Work out the finished part from the listing and answer in its coordinate system (mm). Face numbers are marked on the shaded views. A direction names the side the tool comes from. Round coordinates to 2 decimals unless told otherwise and drop trailing zeros. Write each loop counter-clockwise with the first axis right and the second up, starting at its lowest first coordinate (ties: lowest second). Pieces come first, ordered by that corner, then holes. Notation, with made-up numbers: (27.25, 89.5) - (72.25, 89.5) arc R12 ccw to (72.25, 110.5) - close; hole circle Ø1 at (69, 11). An arc over 180 degrees is marked (long way). Answer as a JSON object with one key per item and string values.
```python
from build123d import *

# Parameters (mm, degrees)
SKETCH1_W                  = 30
SKETCH1_H                  = 30
SKETCH1_R                  = 1.6
SKETCH1_W_2                = 70
SKETCH1_H_2                = 12
BOSS_EXTRUDE1_DEPTH        = 6
SKETCH1_3_W                = 30
SKETCH1_3_H                = 30
SKETCH1_3_R                = 1.6
BOSS_EXTRUDE2_DEPTH        = 22.33
CUT_EXTRUDE1_DEPTH         = 78.612040947
SKETCH3_R                  = 2.55
CUT_EXTRUDE2_DEPTH         = 8
CUT_EXTRUDE3_DEPTH         = 4.5
SKETCH6_R                  = 5
CUT_EXTRUDE5_DEPTH         = 8.6
SKETCH7_R                  = 1.6
CUT_EXTRUDE6_DEPTH         = 101.740403513
SKETCH8_R                  = 2.85
CUT_EXTRUDE7_DEPTH         = 11
BOSS_EXTRUDE3_START        = 2.43
SKETCH9_R                  = 3.4
SKETCH9_R_2                = 2.55
BOSS_EXTRUDE3_DEPTH        = 2.43
CHAMFER1_SIZE              = 1.2
FILLET3_R                  = 4
CHAMFER2_SIZE              = 0.8
CUT_EXTRUDE8_DEPTH         = 3
CHAMFER3_SIZE              = 0.8
LPATTERN1_COUNT            = 3
LPATTERN1_PITCH            = 25
CHAMFER3_OF_LPATTERN1_SIZE = 0.8
SKETCH12_W                 = 103.210606925
SKETCH12_H                 = 33.832940417
CUT_EXTRUDE9_DEPTH         = 6


with BuildPart() as part:
    # Sketch1 → Boss-Extrude1 (new body)
    # profile 1 of 2: a face of its own
    with BuildSketch(Plane.XY):
        with Locations((10, 10)):
            Rectangle(SKETCH1_W, SKETCH1_H)
        with Locations((20, 0)):
            Circle(SKETCH1_R, mode=Mode.SUBTRACT)
        with Locations((20, 20)):
            Circle(SKETCH1_R, mode=Mode.SUBTRACT)
        with Locations((0, 20)):
            Circle(SKETCH1_R, mode=Mode.SUBTRACT)
        Circle(SKETCH1_R, mode=Mode.SUBTRACT)
    # profile 2 of 2: a face of its own
    with BuildSketch(Plane.XY):
        with Locations((60, 10)):
            Rectangle(SKETCH1_W_2, SKETCH1_H_2)
    extrude(amount=BOSS_EXTRUDE1_DEPTH)

    # Sketch1<3> → Boss-Extrude2 (add)
    with BuildSketch(Plane.XY):
        with Locations((10, 10)):
            Rectangle(SKETCH1_3_W, SKETCH1_3_H)
        with Locations((20, 0)):
            Circle(SKETCH1_3_R, mode=Mode.SUBTRACT)
        with Locations((20, 20)):
            Circle(SKETCH1_3_R, mode=Mode.SUBTRACT)
        with Locations((0, 20)):
            Circle(SKETCH1_3_R, mode=Mode.SUBTRACT)
        Circle(SKETCH1_3_R, mode=Mode.SUBTRACT)
    extrude(amount=BOSS_EXTRUDE2_DEPTH)

    # Sketch2 → Cut-Extrude1 (cut, through all)
    with BuildSketch(Plane(origin=(25, 0, 0), x_dir=(0, 0, -1), z_dir=(1, 0, 0))):
        with BuildLine():
            Line((-6.515476918, 16.231667643), (-9.112158418, 16.231667643))
            Line((-9.112158418, 16.231667643), (-10.20449761, 16.039058771))
            ThreePointArc((-10.20449761, 16.039058771), (-11.275650893, 14.693383456), (-12.742453793, 15.59154862))
            Line((-12.742453793, 15.59154862), (-13.786185118, 15.407510627))
            Line((-13.786185118, 15.407510627), (-13.786185118, 4.591753459))
            Line((-13.786185118, 4.591753459), (-12.742453793, 4.407715465))
            ThreePointArc((-12.742453793, 4.407715465), (-11.275650893, 5.305880629), (-10.20449761, 3.960205314))
            Line((-10.20449761, 3.960205314), (-9.112158418, 3.767596443))
            Line((-9.112158418, 3.767596443), (-6.515476918, 3.767596443))
            Line((-6.515476918, 3.767596443), (-5.902540869, 3.767596443))
            Line((-5.902540869, 3.767596443), (-5.902540869, 16.231667643))
            Line((-5.902540869, 16.231667643), (-6.515476918, 16.231667643))
        make_face()
    extrude(amount=-CUT_EXTRUDE1_DEPTH, mode=Mode.SUBTRACT)

    # Sketch3 → Cut-Extrude2 (cut)
    with BuildSketch(Plane.XY.offset(22.33)):
        with Locations((10, 10)):
            Circle(SKETCH3_R)
    extrude(amount=-CUT_EXTRUDE2_DEPTH, mode=Mode.SUBTRACT)

    # Sketch5 → Cut-Extrude3 (cut)
    with BuildSketch(Plane(origin=(0, 0, 13.786185118), x_dir=(-1, 0, 0), z_dir=(0, 0, -1))):
        Polygon((-5.32346282, 10), (-7.66173141, 14.05), (-12.33826859, 14.05), (-14.67653718, 10), (-12.33826859, 5.95), (-7.66173141, 5.95), align=None)
    extrude(amount=-CUT_EXTRUDE3_DEPTH, mode=Mode.SUBTRACT)

    # Sketch6 → Cut-Extrude5 (cut)
    with BuildSketch(Plane(origin=(0, 0, 0), x_dir=(-1, 0, 0), z_dir=(0, 0, -1))):
        with Locations((-10, 10)):
            Circle(SKETCH6_R)
    extrude(amount=-CUT_EXTRUDE5_DEPTH, mode=Mode.SUBTRACT)

    # Sketch7 → Cut-Extrude6 (cut, through all)
    with BuildSketch(Plane(origin=(0, 0, 0), x_dir=(-1, 0, 0), z_dir=(0, 0, -1))):
        with BuildLine():
            ThreePointArc((-90.1, 10), (-88.5, 8.4), (-86.9, 10))
            Line((-86.9, 10), (-90.1, 10))
        make_face()
        with BuildLine():
            Line((-90.1, 10), (-86.9, 10))
            ThreePointArc((-86.9, 10), (-88.5, 11.6), (-90.1, 10))
        make_face()
        with Locations((-63.5, 10)):
            Circle(SKETCH7_R)
        with Locations((-38.5, 10)):
            Circle(SKETCH7_R)
    extrude(amount=-CUT_EXTRUDE6_DEPTH, mode=Mode.SUBTRACT)

    # Sketch8 → Cut-Extrude7 (cut)
    with BuildSketch(Plane.XY.offset(22.33)):
        with Locations((20, 20)):
            Circle(SKETCH8_R)
        with Locations((20, 0)):
            Circle(SKETCH8_R)
        Circle(SKETCH8_R)
        with Locations((0, 20)):
            Circle(SKETCH8_R)
    extrude(amount=-CUT_EXTRUDE7_DEPTH, mode=Mode.SUBTRACT)

    # Sketch9 → Boss-Extrude3 (add)
    with BuildSketch(Plane.XY.offset(22.33).offset(BOSS_EXTRUDE3_START)):
        with Locations(Location((10, 10, 0), (0, 0, 180))):
            Circle(SKETCH9_R)
        with Locations((10, 10)):
            Circle(SKETCH9_R_2, mode=Mode.SUBTRACT)
    extrude(amount=-BOSS_EXTRUDE3_DEPTH)

    # Chamfer1
    chamfer1_edges = [part.edges().sort_by_distance(p)[0] for p in [
        (13.4, 10, 22.33),
    ]]
    chamfer(chamfer1_edges, length=CHAMFER1_SIZE)

    # Fillet3
    # the kernel refuses this fillet: 4 mm, written as the material it adds along each edge
    with BuildSketch(Plane(origin=(25, 4, 0), x_dir=(0, -1, 0), z_dir=(0, 0, 1))) as fillet3_piece_1:
        with BuildLine():
            CenterArc((FILLET3_R, FILLET3_R), FILLET3_R, 180, 90)
            Line((0, FILLET3_R), (0, 0))
            Line((0, 0), (FILLET3_R, 0))
        make_face()
    extrude(amount=5.902540869)
    with BuildSketch(Plane(origin=(25, 16, 0), x_dir=(0, 1, 0), z_dir=(0, 0, 1))) as fillet3_piece_2:
        with BuildLine():
            CenterArc((FILLET3_R, -FILLET3_R), FILLET3_R, 90, 90)
            Line((0, -FILLET3_R), (0, 0))
            Line((0, 0), (FILLET3_R, 0))
        make_face()
    extrude(amount=5.902540869)
    # the kernel refuses this fillet: 4 mm, written as the material it takes off along each edge
    with BuildSketch(Plane(origin=(-5, -5, 32.33), x_dir=(1, 0, 0), z_dir=(0, 0, -1)), Plane(origin=(-5, 25, 32.33), x_dir=(0, -1, 0), z_dir=(0, 0, -1)), Plane(origin=(25, 25, -10), x_dir=(0, -1, 0), z_dir=(0, 0, 1)), Plane(origin=(25, -5, -10), x_dir=(-1, 0, 0), z_dir=(0, 0, 1))) as fillet3_2_piece_1:
        with BuildLine():
            CenterArc((FILLET3_R, -FILLET3_R), FILLET3_R, 90, 90)
            Line((0, -FILLET3_R), (0, 0))
            Line((0, 0), (FILLET3_R, 0))
        make_face()
    extrude(amount=42.33, mode=Mode.SUBTRACT)
    with BuildSketch(Plane(origin=(95, 16, -10), x_dir=(-1, 0, 0), z_dir=(0, 0, 1))) as fillet3_2_piece_2:
        with BuildLine():
            CenterArc((FILLET3_R, FILLET3_R), FILLET3_R, 180, 90)
            Line((0, FILLET3_R), (0, 0))
            Line((0, 0), (FILLET3_R, 0))
        make_face()
    extrude(amount=26, mode=Mode.SUBTRACT)
    with BuildSketch(Plane(origin=(95, 4, -10), x_dir=(-1, 0, 0), z_dir=(0, 0, 1))) as fillet3_2_piece_3:
        with BuildLine():
            CenterArc((FILLET3_R, -FILLET3_R), FILLET3_R, 90, 90)
            Line((0, -FILLET3_R), (0, 0))
            Line((0, 0), (FILLET3_R, 0))
        make_face()
    extrude(amount=26, mode=Mode.SUBTRACT)

    # Chamfer2
    chamfer2_edges = [part.edges().sort_by_distance(p)[0] for p in [
        (-2.85, 20, 22.33),
        (-2.85, 0, 22.33),
        (17.15, 0, 22.33),
        (17.15, 20, 22.33),
    ]]
    chamfer(chamfer2_edges, length=CHAMFER2_SIZE)

    # Sketch10 → Cut-Extrude8 (cut)
    with BuildSketch(Plane(origin=(0, 0, 0), x_dir=(-1, 0, 0), z_dir=(0, 0, -1))):
        Polygon((-85.266838493, 10), (-86.883419246, 12.8), (-90.116580754, 12.8), (-91.733161507, 10), (-90.116580754, 7.2), (-86.883419246, 7.2), align=None)
    cut_extrude8 = extrude(amount=-CUT_EXTRUDE8_DEPTH, mode=Mode.SUBTRACT)

    # Chamfer3
    chamfer3_edges = [part.edges().sort_by_distance(p)[0] for p in [
        (86.075128869, 8.6, 0),
        (86.075128869, 11.4, 0),
        (88.5, 12.8, 0),
        (90.924871131, 11.4, 0),
        (90.924871131, 8.6, 0),
        (88.5, 7.2, 0),
    ]]
    chamfer(chamfer3_edges, length=CHAMFER3_SIZE)

    # LPattern1: Cut-Extrude8 ×3
    with Locations(*[(-i * LPATTERN1_PITCH, 0, 0) for i in range(1, LPATTERN1_COUNT)]):
        add(cut_extrude8, mode=Mode.SUBTRACT)

    # Chamfer3 of LPattern1
    chamfer3_of_lpattern1_edges = [part.edges().sort_by_distance(p)[0] for p in [
        (61.075128869, 8.6, 0),
        (61.075128869, 11.4, 0),
        (63.5, 12.8, 0),
        (65.924871131, 11.4, 0),
        (65.924871131, 8.6, 0),
        (63.5, 7.2, 0),
        (36.075128869, 8.6, 0),
        (36.075128869, 11.4, 0),
        (38.5, 12.8, 0),
        (40.924871131, 11.4, 0),
        (40.924871131, 8.6, 0),
        (38.5, 7.2, 0),
    ]]
    chamfer(chamfer3_of_lpattern1_edges, length=CHAMFER3_OF_LPATTERN1_SIZE)

    # Sketch12 → Cut-Extrude9 (cut)
    with BuildSketch(Plane(origin=(0, 0, 0), x_dir=(-1, 0, 0), z_dir=(0, 0, -1))):
        with Locations((-45.050346637, 9.848960088)):
            Rectangle(SKETCH12_W, SKETCH12_H)
    extrude(amount=-CUT_EXTRUDE9_DEPTH, mode=Mode.SUBTRACT)


solid = part.part
```
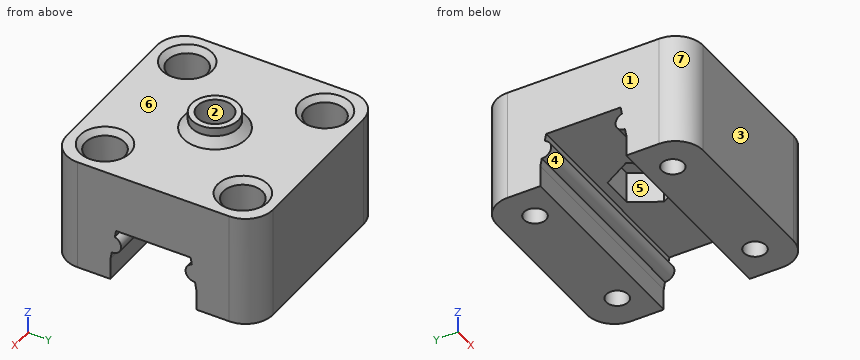
Item 1: A cutting plane is placed at B-B (x = 20). Give the number of separate pieces and of enclosed holes in the cut face, and give its area (3 significant figures).
Results found:
{"separate pieces": "3", "enclosed holes": "0", "area": "240 mm²"}
Item 2: Determine the mould class of the marked faces 1, 2 and 3 for opening direction Y: pulls with the +Y half, pulls with the -Y half, needs draft (parallel to the pull), parting line crosses it, or undercut.
Results found:
{"face 1": "needs draft", "face 2": "undercut", "face 3": "pulls with the -Y half"}
Item 3: A cutting plane is placed at C-C (y = 0). Write down the section's boundary in (x, z).
Results found:
{"outline": "(-5, 6) - (-1.6, 6) - (-1.6, 11.33) - (-2.85, 11.33) - (-2.85, 21.53) - (-3.65, 22.33) - (-5, 22.33) - close; (1.6, 6) - (18.4, 6) - (18.4, 11.33) - (17.15, 11.33) - (17.15, 21.53) - (16.35, 22.33) - (3.65, 22.33) - (2.85, 21.53) - (2.85, 11.33) - (1.6, 11.33) - close; (21.6, 6) - (25, 6) - (25, 22.33) - (23.65, 22.33) - (22.85, 21.53) - (22.85, 11.33) - (21.6, 11.33) - close"}
Item 4: A cutting plane is placed at D-D (x = 10). Write down the section's boundary in (y, z), and give its area (3 significant figures).
Results found:
{"outline": "(-5, 6) - (3.77, 6) - (3.77, 9.11) - (3.96, 10.2) arc R1.3 ccw to (4.41, 12.74) - (4.59, 13.79) - (5.95, 13.79) - (5.95, 18.29) - (7.45, 18.29) - (7.45, 24.76) - (6.6, 24.76) - (6.6, 23.53) - (5.4, 22.33) - (-5, 22.33) - close; (12.55, 18.29) - (14.05, 18.29) - (14.05, 13.79) - (15.41, 13.79) - (15.59, 12.74) arc R1.3 ccw to (16.04, 10.2) - (16.23, 9.11) - (16.23, 6) - (25, 6) - (25, 22.33) - (14.6, 22.33) - (13.4, 23.53) - (13.4, 24.76) - (12.55, 24.76) - close", "area": "350 mm²"}
Item 5: A cutting plane is placed at A-A (z = 7.75). Write down the section's boundary in (x, y).
Results found:
{"outline": "(-5, -1) arc R4 ccw to (-1, -5) - (21, -5) arc R4 ccw to (25, -1) - (25, 3.77) - (-5, 3.77) - close; (-5, 16.23) - (25, 16.23) - (25, 21) arc R4 ccw to (21, 25) - (-1, 25) arc R4 ccw to (-5, 21) - close; hole circle Ø3.2 at (0, 0); hole circle Ø3.2 at (0, 20); hole circle Ø3.2 at (20, 0); hole circle Ø3.2 at (20, 20)"}
Item 6: For the marked faces 4, 5, 6 and 7, determine the directions among +Z, -Z, +X, -X, +Y, -Y from which every point of the face is accessible in a straight line to the end or side of a thin tool.
Results found:
{"face 4": "+X, -X", "face 5": "-Z", "face 6": "+Z", "face 7": "+Z, -Z, -X, -Y"}
Item 7: Each of these flat-tipped pins is pushed along its axis until it touches: P1, Ø2, axis at x = 12.5, y = 11.5, coming from the -Z side; P2, Ø4, axis at x = 15, y = 3.5, coming from the +Z side; P3, Ø6.5, axis at x = 9, y = 9.5, coming from the -Z side. Where does it stop, or does it pass through?
Results found:
{"P1": "z = 18.29", "P2": "z = 22.33", "P3": "z = 13.79"}
Item 8: Consider line 1 along X through (y, z) = (0, 9.55); line 2 along Y through (x, z) = (0, 18.5); line 3 along Y through (x, z) = (8, 7). Determine where each line is inside the solid, lowest interval first.
Results found:
{"line 1": "-5 to -1.6, 1.6 to 18.4, 21.6 to 25", "line 2": "-5 to -2.85, 2.85 to 17.15, 22.85 to 25", "line 3": "-5 to 3.77, 16.23 to 25"}
